For this review, take the finished solid that the model builds, in its own axes (mm). Round coordinates to 2 decimals unless told otherwise and drop trailing zeros. Loops run counter-clockwise (first coordinate to the right, second up) from the corner with the lowest first, then second, coordinate; pieces in that order, holes last.
```python
from build123d import *

# Parameters (mm, degrees)
F0_W     = 19.05
F0_H     = 101.6
F1_DEPTH = 63.5
F3_R     = 31.75
F4_DEPTH = 19.05
F6_R     = 1.5875
F7_DEPTH = 63.5
F8_R     = 5.08


with BuildPart() as f1:
    # F0 (on Front) → F1 (new body)
    with BuildSketch(Plane.XZ):
        Rectangle(F0_W, F0_H)
    extrude(amount=F1_DEPTH)

    # F3 (on offset) → F4 (cut)
    with BuildSketch(Plane(origin=(-9.525, 0, 0), x_dir=(0, -1, 0), z_dir=(-1, 0, 0))):
        with Locations((63.5, 0)):
            Circle(F3_R)
    extrude(amount=-F4_DEPTH, mode=Mode.SUBTRACT)

    # F6 (on offset) → F7 (cut)
    with BuildSketch(Plane.XZ.offset(63.5)):
        with Locations((0, 41.275)):
            Circle(F6_R)
        with Locations((0, -41.275)):
            Circle(F6_R)
    extrude(amount=-F7_DEPTH, mode=Mode.SUBTRACT)

    # F8
    f8_edges = [f1.edges().sort_by_distance(p)[0] for p in [
        (-9.525, -31.75, 50.8),
        (-9.525, -31.75, -50.8),
        (9.525, -31.75, -50.8),
        (9.525, -31.75, 50.8),
    ]]
    fillet(f8_edges, radius=F8_R)


solid = f1.part
```
(1) Add section A-A (x = 0). Give the boundary of the cut face in (y, z), plus the area to 3 significant figures.
(2) Add section B-B (y = -58). Give the boundary of the cut face in (x, z) (1 decimal).
(3) Add section D-D (y = -7). Give the boundary of the cut face in (x, z) (1 decimal).
(4) Insertion check: pin 1 Ø3 at (x, y) = (-7.5, -49) entering from -Z; pin 2 Ø2.5 at (x, z) = (0, 41.275) entering from +Y; pin 3 Ø4 at (x, z) = (6, 14) entering from +Y. Each pin has a flat end and moves straight along its axis. Give the tip position at first contact, or say it passes through.
(5) For L1, parallel to Z at x = 0, y = -26.5; L2, parallel to Z at x = 0, y = -50; L3, parallel to Z at x = 0, y = -48.5, list the stretches that pass through material, from the lowest coordinate up.
(6) Add section C-C (z = 0). Give the boundary of the cut face in (x, y) (3 decimals), plus the area to 3 significant figures.
(7) The part is to be moulded in two halves that separate along Z. For faces 1 (the flat face through (0, -31, 50.8)), 2 (the cylindrical face through (-8.08, -32.19, -49.27)), 3 (the cylindrical face through (-0.344, -32.194, 39.725)), say which applies: pulls with the +Z half, pulls with the -Z half, needs draft (parallel to the pull), parting line crosses it, or undercut.
Outcome:
1. outline: (-63.5, -50.8) - (0, -50.8) - (0, -42.86) - (-63.5, -42.86) - close; (-63.5, -39.69) - (0, -39.69) - (0, 39.69) - (-63.5, 39.69) - (-63.5, 31.75) arc R31.75 cw to (-63.5, -31.75) - close; (-63.5, 42.86) - (0, 42.86) - (0, 50.8) - (-63.5, 50.8) - close
1. area: 4,460 mm2
2. outline: (-9.5, -45.7) arc R5.1 ccw to (-4.4, -50.8) - (4.4, -50.8) arc R5.1 ccw to (9.5, -45.7) - (9.5, -31.3) - (-9.5, -31.3) - close; (-9.5, 31.3) - (9.5, 31.3) - (9.5, 45.7) arc R5.1 ccw to (4.4, 50.8) - (-4.4, 50.8) arc R5.1 ccw to (-9.5, 45.7) - close; hole circle Ø3.2 at (0, -41.3); hole circle Ø3.2 at (0, 41.3)
3. outline: (-9.5, -45.7) arc R5.1 ccw to (-4.4, -50.8) - (4.4, -50.8) arc R5.1 ccw to (9.5, -45.7) - (9.5, 45.7) arc R5.1 ccw to (4.4, 50.8) - (-4.4, 50.8) arc R5.1 ccw to (-9.5, 45.7) - close; hole circle Ø3.2 at (0, -41.3); hole circle Ø3.2 at (0, 41.3)
4. pin 1: stops at z = -50.56
4. pin 2: passes through
4. pin 3: stops at y = 0
5. L1: z = -50.8 to -42.86, -39.69 to 39.69, 42.86 to 50.8
5. L2: z = -50.8 to -42.86, -39.69 to -28.74, 28.74 to 39.69, 42.86 to 50.8
5. L3: z = -50.8 to -42.86, -39.69 to -27.98, 27.98 to 39.69, 42.86 to 50.8
6. outline: (-9.525, -31.75) - (9.525, -31.75) - (9.525, 0) - (-9.525, 0) - close
6. area: 605 mm2
7. face 1: pulls with the +Z half
7. face 2: pulls with the -Z half
7. face 3: undercut
